from build123d import *

# Parameters (mm, degrees)
SKETCH1_R           = 43
BOSS_EXTRUDE2_DEPTH = 3
SKETCH1_3_R         = 3
CUT_EXTRUDE1_DEPTH  = 4
CIRPATTERN2_COUNT   = 6


with BuildPart() as part:
    # Sketch1 → Boss-Extrude2 (new body)
    with BuildSketch(Plane.XY):
        Circle(SKETCH1_R)
    extrude(amount=BOSS_EXTRUDE2_DEPTH)

    # Sketch1_3 → Cut-Extrude1 (cut, through all)
    with BuildSketch(Plane.XY):
        with Locations((0, 33)):
            Circle(SKETCH1_3_R)
    cut_extrude1 = extrude(amount=CUT_EXTRUDE1_DEPTH, mode=Mode.SUBTRACT)

    # CirPattern2: Cut-Extrude1 ×6 about axis
    cirpattern2_axis = Axis((0, 0, 0), (0, 0, 1))
    for i in range(1, CIRPATTERN2_COUNT):
        add(cut_extrude1.rotate(cirpattern2_axis, i * 360 / CIRPATTERN2_COUNT), mode=Mode.SUBTRACT)


solid = part.part
Here's how the part is built. I have some questions about the finished solid (model axes, mm). Coordinates: 2 decimals unless noted, no trailing zeros. Write each loop counter-clockwise with the first axis right and the second up, starting at its lowest first coordinate (ties: lowest second). Pieces come first, ordered by that corner, then holes.
Item 1: Will these pins go through, and if not, where does the flat tip stop? pin 1 (12 mm diameter, centred on x = -16, y = -11.5, fed in from -Z); pin 2 (3.5 mm diameter, centred on x = -28.58, y = -16.5, fed in from -Z).
Item 2: I want a section at C-C on z = 1.05. Write out the boundary of the cut face in (x, y).
Item 3: I want a section at A-A on x = 0. Write out the boundary of the cut face in (y, z), and give its area (3 significant figures).
Item 4: I want a section at B-B on y = 16. Write out the boundary of the cut face in (x, z), and give its area (3 significant figures).
Item 5: I want a section at D-D on y = -33. Write out the boundary of the cut face in (x, z).
Item 6: If I drill on line 1 (Y direction, x = 0, z = 1.5); line 2 (Y direction, x = 28, z = 1.45); line 3 (X direction, y = -16, z = 1.5), over which ranges is the centre line in solid material (lowest first)?
Item 7: If we mould it in two halves opening along Y, with no side actions, what happens to faces 1 (the flat face through (-1, 1, 0)), 2 (the cylindrical face through (-5.598, 42.634, 1.479)), 3 (the cylindrical face through (25.81, 17.65, 1.48)), 4 (the cylindrical face through (-25.81, -17.65, 1.48))? For each: +Y half, -Y half, draft (parallel to the pull), parting line (faces both ways), or undercut.
Findings below:
1. pin 1: stops at z = 0
1. pin 2: passes through
2. outline: circle Ø86 at (0, 0); hole circle Ø6 at (-28.58, -16.5); hole circle Ø6 at (-28.58, 16.5); hole circle Ø6 at (0, -33); hole circle Ø6 at (0, 33); hole circle Ø6 at (28.58, -16.5); hole circle Ø6 at (28.58, 16.5)
3. outline: (-43, 0) - (-36, 0) - (-36, 3) - (-43, 3) - close; (-30, 0) - (30, 0) - (30, 3) - (-30, 3) - close; (36, 0) - (43, 0) - (43, 3) - (36, 3) - close
3. area: 222 mm2
4. outline: (-39.91, 0) - (-31.54, 0) - (-31.54, 3) - (-39.91, 3) - close; (-25.62, 0) - (25.62, 0) - (25.62, 3) - (-25.62, 3) - close; (31.54, 0) - (39.91, 0) - (39.91, 3) - (31.54, 3) - close
4. area: 204 mm2
5. outline: (-27.57, 0) - (-3, 0) - (-3, 3) - (-27.57, 3) - close; (3, 0) - (27.57, 0) - (27.57, 3) - (3, 3) - close
6. line 1: y = -43 to -36, -30 to 30, 36 to 43
6. line 2: y = -32.63 to -19.44, -13.56 to 13.56, 19.44 to 32.63
6. line 3: x = -39.91 to -31.54, -25.62 to 25.62, 31.54 to 39.91
7. face 1: draft
7. face 2: parting line
7. face 3: undercut
7. face 4: undercut
